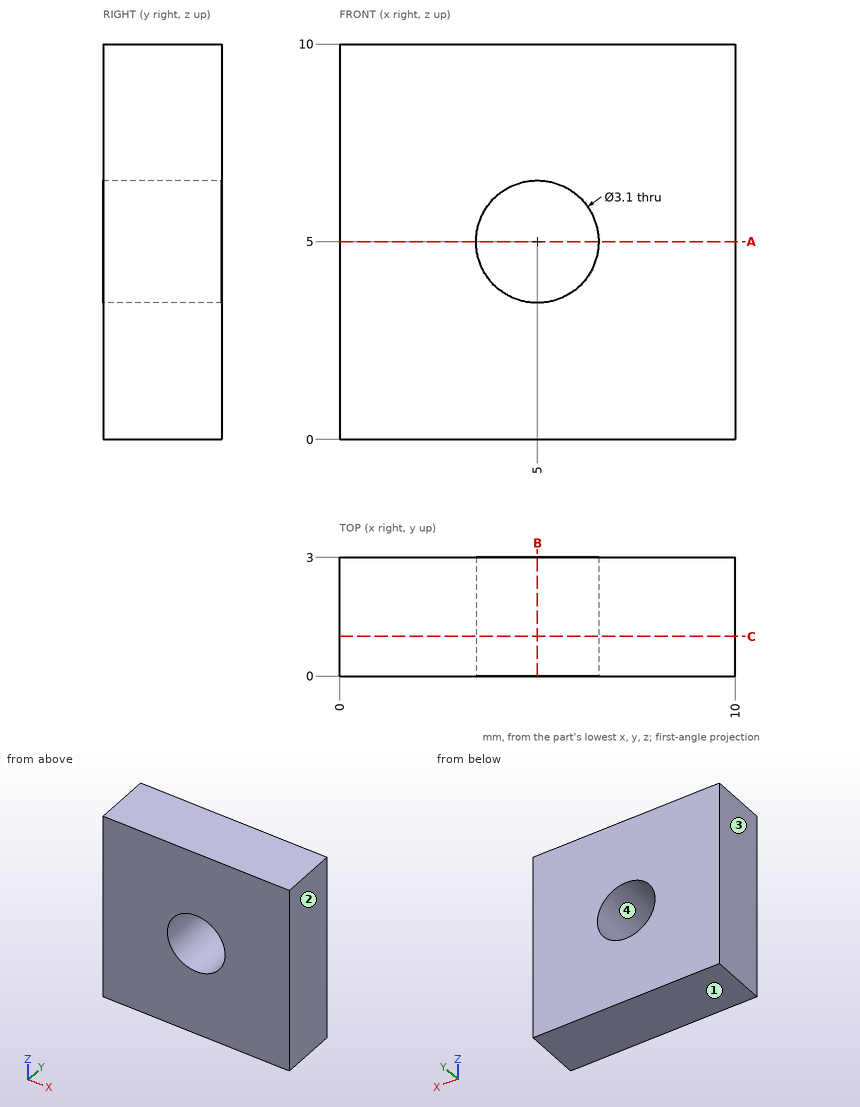
Here's the drawing with two shaded views (mm, measured from the low corner). I have some questions. Coordinates: 2 decimals unless noted, no trailing zeros. Order: outer loops, then holes, each group sorted by start corner. A loop starts at its lowest first (then second) coordinate and runs counter-clockwise, first axis right, second up.
Item 1: I need wall thicknesses on line 1 (X direction, y = 1.7, z = 5); line 2 (X direction, y = 0.9, z = 4.25). Which ranges of each line are inside material? Lowest first, please.
Result sheet:
line 1: x = 0 to 3.45, 6.55 to 10
line 2: x = 0 to 3.64, 6.36 to 10
Item 2: If we section it at C-C on y = 1: List the corners of the cut face in (x, z) for me.
Result sheet:
outline: (0, 0) - (10, 0) - (10, 10) - (0, 10) - close; hole circle Ø3.1 at (5, 5)
Item 3: If we mould it in two halves opening along X, with no side actions, what happens to the marked faces 1, 2, 3 and 4? For each: +X half, -X half, draft (parallel to the pull), parting line (faces both ways), or undercut.
Result sheet:
face 1: draft
face 2: +X half
face 3: -X half
face 4: undercut
Item 4: If we section it at B-B on x = 5: List the corners of the cut face in (y, z) for me, plus the area to 3 significant figures.
Result sheet:
outline: (0, 0) - (3, 0) - (3, 3.45) - (0, 3.45) - close; (0, 6.55) - (3, 6.55) - (3, 10) - (0, 10) - close
area: 20.7 mm2
Item 5: If we section it at A-A on z = 5: List the corners of the cut face in (x, y) for me, plus the area to 3 significant figures.
Result sheet:
outline: (0, 0) - (3.45, 0) - (3.45, 3) - (0, 3) - close; (6.55, 0) - (10, 0) - (10, 3) - (6.55, 3) - close
area: 20.7 mm2
